For this review, take the finished solid that the model builds, in its own axes (mm). A direction names the side the tool comes from. Give positions to 0.01 mm unless a question says otherwise; leave off trailing zeros. Loops run counter-clockwise (first coordinate to the right, second up) from the corner with the lowest first, then second, coordinate; pieces in that order, holes last. Notation, with made-up numbers: M 4,14.25 L 60,14.25 A36 ccw 60,53.25 Z; hole C -38,83 d8. An arc over 180 degrees is marked long. Use CSV: the item, a comma, the result in double quotes. Start each with the question number.
1. Insertion check: P1, Ø1.6, axis at y = 1.5, z = 17.5, coming from the -X side; P2, Ø5, axis at x = 0, y = 30, coming from the -Z side; P3, Ø4, axis at x = -20, z = -3, coming from the +Y side; P4, Ø4, axis at y = 8, z = -4.5, coming from the +X side. Each pin has a flat end and moves straight along its axis. Give the tip position at first contact, or say it passes through.
2. Take a section at C-C, the plane y = 30. Write out the cut boundary in (x, z), and give its area (3 significant figures).
3. Tool access review of faces 1 (the face through (37, 3, 17)), 2 (the face through (35, 2, -11.5)), 3 (the face through (-25.944, 1.972, 5.67)), 4 (the face through (-37, 1, -17)): name each direction out of +Z, -Z, +X, -X, +Y, -Y from which nothing blocks a thin tool from reaching the whole face with its end or side.
4. To check wall thickness, follow line 1 (Y direction, x = 0, z = -1); line 2 (X direction, y = 30, z = -0.25); line 3 (Y direction, x = 34, z = -16.5). State the ranges of each line that lie inside material, in increasing order. Write a range as [from, to].
5. Take a section at A-A, the plane z = -15.5. Write out the cut boundary in (x, y).
6. Take a section at D-D, the plane z = 19. Write out the cut boundary in (x, y) (3 decimals).
7. The part is to be moulded in two halves that separate along Y. For faces 5 (the face through (-1, 0, 0)), 6 (the face through (-37, 2, -13.5)), 7 (the face through (36, 2, -22.5)), 8 (the face through (1.847, 29.234, 0.056)), say which applies: pulls with the +Y half, pulls with the -Y half, needs draft (parallel to the pull), parting line crosses it, or undercut.
8. Take a section at B-B, the plane x = -27. Write out the cut boundary in (y, z).
from build123d import *

# Parameters (mm, degrees)
SALIENTE_EXTRUIR1_DEPTH    = 4
CROQUIS4_W                 = 7
CROQUIS4_H                 = 2
CORTAR_EXTRUIR2_DEPTH      = 9
CROQUIS6_W                 = 7
CROQUIS6_H                 = 2
CORTAR_EXTRUIR6_DEPTH      = 9
CROQUIS7_W                 = 7
CROQUIS7_H                 = 2
CORTAR_EXTRUIR4_DEPTH      = 9
CROQUIS8_W                 = 7
CROQUIS8_H                 = 2
CORTAR_EXTRUIR5_DEPTH      = 9
CROQUIS9_R                 = 4
SALIENTE_EXTRUIR2_DEPTH    = 30
CROQUIS10_R                = 2
CORTAR_EXTRUIR7_DEPTH      = 23.5
CORTAR_EXTRUIR7_DEPTH_BACK = 23.5


with BuildPart() as part:
    # Croquis1 → Saliente-Extruir1 (new body)
    with BuildSketch(Plane(origin=(0, 0, 0), x_dir=(1, 0, 0), z_dir=(0, 1, 0))):
        Polygon((-41, -22.5), (-30, -22.5), (0, -14.5), (30, -22.5), (41, -22.5), (41, -11.5), (30, -11.5), (22, 0), (30, 11.5), (41, 11.5), (41, 22.5), (30, 22.5), (0, 14.5), (-30, 22.5), (-41, 22.5), (-41, 11.5), (-30, 11.5), (-22, 0), (-30, -11.5), (-41, -11.5), align=None)
    extrude(amount=SALIENTE_EXTRUIR1_DEPTH)

    # Croquis4 → Cortar-Extruir2 (cut)
    with BuildSketch(Plane.ZY.offset(41)):
        with Locations((-17, 2)):
            Rectangle(CROQUIS4_W, CROQUIS4_H)
    extrude(amount=-CORTAR_EXTRUIR2_DEPTH, mode=Mode.SUBTRACT)

    # Croquis6 → Cortar-Extruir6 (cut)
    with BuildSketch(Plane.ZY.offset(41)):
        with Locations((17, 2)):
            Rectangle(CROQUIS6_W, CROQUIS6_H)
    extrude(amount=-CORTAR_EXTRUIR6_DEPTH, mode=Mode.SUBTRACT)

    # Croquis7 → Cortar-Extruir4 (cut)
    with BuildSketch(Plane(origin=(41, 0, 0), x_dir=(0, 0, -1), z_dir=(1, 0, 0))):
        with Locations((-17, 2)):
            Rectangle(CROQUIS7_W, CROQUIS7_H)
    extrude(amount=-CORTAR_EXTRUIR4_DEPTH, mode=Mode.SUBTRACT)

    # Croquis8 → Cortar-Extruir5 (cut)
    with BuildSketch(Plane(origin=(41, 0, 0), x_dir=(0, 0, -1), z_dir=(1, 0, 0))):
        with Locations((17, 2)):
            Rectangle(CROQUIS8_W, CROQUIS8_H)
    extrude(amount=-CORTAR_EXTRUIR5_DEPTH, mode=Mode.SUBTRACT)

    # Croquis9 → Saliente-Extruir2 (add)
    with BuildSketch(Plane(origin=(0, 4, 0), x_dir=(1, 0, 0), z_dir=(0, 1, 0))):
        Circle(CROQUIS9_R)
    extrude(amount=SALIENTE_EXTRUIR2_DEPTH)

    # Croquis10 → Cortar-Extruir7 (cut, two sides)
    with BuildSketch(Plane.XY) as cortar_extruir7_sk:
        with Locations((0, 30)):
            Circle(CROQUIS10_R)
    extrude(amount=CORTAR_EXTRUIR7_DEPTH, mode=Mode.SUBTRACT)
    extrude(cortar_extruir7_sk.sketch, amount=-CORTAR_EXTRUIR7_DEPTH_BACK, mode=Mode.SUBTRACT)


solid = part.part
Result set:
1,P1,"x = -41"
1,P2,"z = -4"
1,P3,"y = 4"
1,P4,"x = 3.12"
2,outline,"M -2,-3.46 L -2,3.46 A4 ccw Z; M 2,-3.46 A4 ccw 2,3.46 Z"
2,area,"19.7 mm2"
3,face 1,"+X"
3,face 2,"+X, +Y, -Y"
3,face 3,"-X, +Y, -Y"
3,face 4,"-X"
4,line 1,"[0, 28], [32, 34]"
4,line 2,"[-3.99, -2], [2, 3.99]"
4,line 3,"[0, 1], [3, 4]"
5,outline,"M -41,0 L -3.75,0 L -3.75,4 L -41,4 L -41,3 L -32,3 L -32,1 L -41,1 Z; M 3.75,0 L 41,0 L 41,1 L 32,1 L 32,3 L 41,3 L 41,4 L 3.75,4 Z"
6,outline,"M -41,0 L -16.875,0 L -16.875,4 L -41,4 L -41,3 L -32,3 L -32,1 L -41,1 Z; M 16.875,0 L 41,0 L 41,1 L 32,1 L 32,3 L 41,3 L 41,4 L 16.875,4 Z"
7,face 5,"pulls with the -Y half"
7,face 6,"undercut"
7,face 7,"needs draft"
7,face 8,"undercut"
8,outline,"M 0,-21.7 L 4,-21.7 L 4,-7.19 L 0,-7.19 Z; M 0,7.19 L 4,7.19 L 4,21.7 L 0,21.7 Z"
